Design review of the part built by this model. Coordinates are the model's own, in mm. A direction names the side the tool comes from. Give positions to 0.01 mm unless a question says otherwise; leave off trailing zeros. Loops run counter-clockwise (first coordinate to the right, second up) from the corner with the lowest first, then second, coordinate; pieces in that order, holes last.
from build123d import *

# Parameters (mm, degrees)
BOSS_EXTRUDE1_DEPTH = 10
SKETCH3_R           = 2.1
CUT_EXTRUDE2_DEPTH  = 10
FILLET1_R           = 10
SKETCH4_W           = 30
SKETCH4_H           = 30
BOSS_EXTRUDE2_DEPTH = 5
SKETCH6_R           = 1
CUT_EXTRUDE3_DEPTH  = 5


with BuildPart() as part:
    # Sketch2 → Boss-Extrude1 (new body)
    with BuildSketch(Plane(origin=(0, 0, 0), x_dir=(0, 0, -1), z_dir=(1, 0, 0))):
        Polygon((0, 0), (63, 0), (63, 23.7), (51.5, 23.7), (51.5, 4), (11.5, 4), (11.5, 23.7), (0, 23.7), align=None)
    extrude(amount=BOSS_EXTRUDE1_DEPTH)

    # Sketch3 → Cut-Extrude2 (cut)
    with BuildSketch(Plane(origin=(10, 0, 0), x_dir=(0, 0, -1), z_dir=(1, 0, 0))):
        with Locations((6.738854382, 18.775)):
            Circle(SKETCH3_R)
        with Locations((56.161145618, 18.775)):
            Circle(SKETCH3_R)
        with Locations((56.161145618, 8.925)):
            Circle(SKETCH3_R)
        with Locations((6.738854382, 8.925)):
            Circle(SKETCH3_R)
    extrude(amount=-CUT_EXTRUDE2_DEPTH, mode=Mode.SUBTRACT)

    # Fillet1
    fillet1_edges = [part.edges().sort_by_distance(p)[0] for p in [
        (5, 0, -63),
        (5, 0, 0),
    ]]
    fillet(fillet1_edges, radius=FILLET1_R)

    # Sketch4 → Boss-Extrude2 (add)
    with BuildSketch(Plane.XZ):
        with Locations((3.05, -21.35)):
            Rectangle(SKETCH4_W, SKETCH4_H)
    extrude(amount=BOSS_EXTRUDE2_DEPTH)

    # Sketch6 → Cut-Extrude3 (cut)
    with BuildSketch(Plane.XZ.offset(5)):
        with Locations(Location((-8.45, -8.8, 0), (0, 0, 270))):
            Circle(SKETCH6_R)
        with Locations(Location((12.55, -8.8, 0), (0, 0, 270))):
            Circle(SKETCH6_R)
        with Locations(Location((12.55, -21.3, 0), (0, 0, 270))):
            Circle(SKETCH6_R)
        with Locations(Location((-8.45, -21.3, 0), (0, 0, 270))):
            Circle(SKETCH6_R)
    extrude(amount=-CUT_EXTRUDE3_DEPTH, mode=Mode.SUBTRACT)


solid = part.part
Q1. Take a section at A-A (x = -8.45). Give the boundary of the cut face in (y, z).
Results:
outline: (-5, -36.35) - (0, -36.35) - (0, -22.3) - (-5, -22.3) - close; (-5, -20.3) - (0, -20.3) - (0, -9.8) - (-5, -9.8) - close; (-5, -7.8) - (0, -7.8) - (0, -6.35) - (-5, -6.35) - close
Q2. Take a section at D-D (x = -3.5). Give the boundary of the cut face in (y, z).
Results:
outline: (-5, -36.35) - (0, -36.35) - (0, -6.35) - (-5, -6.35) - close
Q3. Wall thickness on line 1 (X direction, y = -1.6, z = -21.3); line 2 (Z direction, x = 3.25, y = 19.5); line 3 (Z direction, x = 3.25, y = 13): over which ranges is each line inside the solid? List them lowest first.
Results:
line 1: x = -11.95 to -9.45, -7.45 to 11.55, 13.55 to 18.05
line 2: z = -63 to -58.13, -54.19 to -51.5, -11.5 to -8.71, -4.77 to 0
line 3: z = -63 to -51.5, -11.5 to 0
Q4. Insertion check: pin 1 (5 mm diameter, centred on y = 20, z = -54.5, fed in from -X); pin 2 (8 mm diameter, centred on x = 5, z = -28, fed in from +Y); pin 3 (1.6 mm diameter, centred on x = 12.55, z = -8.8, fed in from -Y); pin 4 (1.5 mm diameter, centred on y = 5, z = -9, fed in from +X). Each pin has a flat end and moves straight along its axis. Give the tip position at first contact, or say it passes through.
Results:
pin 1: stops at x = 0
pin 2: stops at y = 4
pin 3: passes through
pin 4: stops at x = 10
Q5. Tool access review of faces 1 (the face through (3, -2, -6.35)), 2 (the face through (5, 23.7, -6)), 3 (the face through (5, 14, -51.5)), 4 (the face through (10, 1, -31)), 5 (the face through (3, -2, -36.35)): name each direction out of +Z, -Z, +X, -X, +Y, -Y from which nothing blocks a thin tool from reaching the whole face with its end or side.
Results:
face 1: +Z, +X, -X, -Y
face 2: +Z, -Z, +X, -X, +Y
face 3: +X, -X, +Y
face 4: +Z, -Z, +X, +Y
face 5: -Z, +X, -X, -Y
Q6. Draft analysis for pull direction X (two halves, no side actions). For faces 6 (the face through (5.07, 16.912, -7.708)), 7 (the face through (-8.4, -2.5, -20.3)), 8 (the face through (0, 1, -31)), 9 (the face through (11.574, -2.535, -21.083)), state which applies: pulls with the +X half, pulls with the -X half, needs draft (parallel to the pull), parting line crosses it, or undercut.
Results:
face 6: needs draft
face 7: undercut
face 8: pulls with the -X half
face 9: undercut
Q7. Take a section at C-C (z = -19.5). Give the boundary of the cut face in (x, y), plus the area to 3 significant figures.
Results:
outline: (-11.95, -5) - (18.05, -5) - (18.05, 0) - (10, 0) - (10, 4) - (0, 4) - (0, 0) - (-11.95, 0) - close
area: 190 mm2
Q8. Take a section at B-B (y = 21.5). Give the boundary of the cut face in (x, z).
Results:
outline: (0, -63) - (10, -63) - (10, -51.5) - (0, -51.5) - close; (0, -11.5) - (10, -11.5) - (10, 0) - (0, 0) - close
